Can you work these out from the model? Positions are in its coordinate system, mm. Face numbers are marked on the shaded views. A direction names the side the tool comes from. Round coordinates to 2 decimals unless told otherwise and drop trailing zeros. Write each loop counter-clockwise with the first axis right and the second up, starting at its lowest first coordinate (ties: lowest second). Pieces come first, ordered by that corner, then holes.
Q1. I'm going to push flat-ended pins straight in: pin 1 Ø5 at (y, z) = (12, 13) entering from +X; pin 2 Ø3 at (y, z) = (5, -2.5) entering from -X; pin 3 Ø5 at (y, z) = (19, 13.5) entering from -X. Where does each tip first touch, or does it pass through?
Q2. If we section it at A-A (y = 11.5): Please give me the cut outline in (x, z).
Q3. Please list where these lines run through material, in increasing order: line 1 along X through (y, z) = (16, 0); line 2 along Y through (x, z) = (19, 3); line 3 along Z through (x, y) = (-10, 17.25).
Q4. We'd pull the mould along X, two halves only. Please class the marked faces 3, 4 and 5: +X half, -X half, draft (parallel to the pull), parting line (faces both ways), or undercut.
Q5. If we section it at B-B (z = -1.5): Please give me the cut outline in (x, y), plus the area to 3 significant figures.
Q6. If we section it at C-C (x = -11.5): Please give me the cut outline in (y, z).
Q7. For the marked faces 1 and 2, which set-ups out of +Z, -Z, +X, -X, +Y, -Y let a thin tool reach every point of the face, with its end or its side?
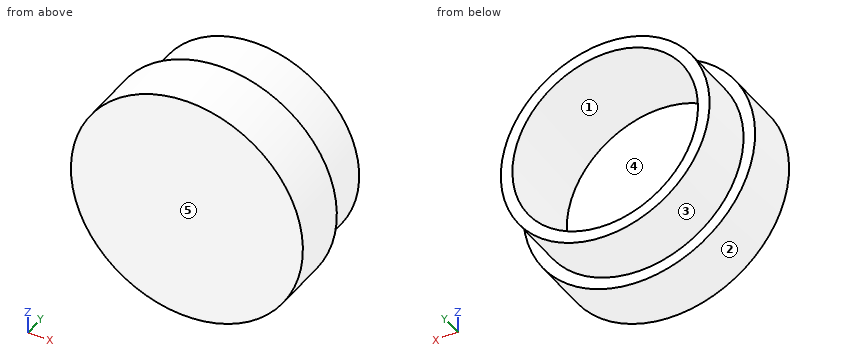
from build123d import *

# Parameters (mm, degrees)
SKETCH1_R           = 25.4
BOSS_EXTRUDE1_DEPTH = 25.4
SHELL2_T            = -5.08
CUT_EXTRUDE3_START  = -12.7
SKETCH3_R           = 25.4
SKETCH3_R_2         = 22.86
CUT_EXTRUDE3_DEPTH  = 12.7


with BuildPart() as part:
    # Sketch1 → Boss-Extrude1 (new body)
    with BuildSketch(Plane(origin=(0, 0, 0), x_dir=(1, 0, 0), z_dir=(0, 1, 0))):
        with Locations(Location((0, 0, 0), (0, 0, 270))):
            Circle(SKETCH1_R)
    extrude(amount=BOSS_EXTRUDE1_DEPTH)

    # Shell2
    shell2_openings = [part.faces().sort_by_distance(p)[0] for p in [
        (0, 25.4, 0),
    ]]
    offset(amount=SHELL2_T, openings=shell2_openings, kind=Kind.INTERSECTION)

    # Sketch3 → Cut-Extrude3 (cut)
    with BuildSketch(Plane(origin=(0, 25.4, 0), x_dir=(1, 0, 0), z_dir=(0, 1, 0)).offset(CUT_EXTRUDE3_START)):
        with Locations(Location((0, 0, 0), (0, 0, 270))):
            Circle(SKETCH3_R)
        with Locations(Location((0, 0, 0), (0, 0, 270))):
            Circle(SKETCH3_R_2, mode=Mode.SUBTRACT)
    extrude(amount=CUT_EXTRUDE3_DEPTH, mode=Mode.SUBTRACT)


solid = part.part
A:
1. pin 1: stops at x = 23.13
1. pin 2: stops at x = -25.38
1. pin 3: stops at x = -20.04
2. outline: circle Ø50.8 at (0, 0); hole circle Ø40.64 at (0, 0)
3. line 1: x = -22.86 to -20.32, 20.32 to 22.86
3. line 2: y = 0 to 5.08
3. line 3: z = -20.56 to -17.69, 17.69 to 20.56
4. face 3: parting line
4. face 4: undercut
4. face 5: draft
5. outline: (-25.36, 0) - (25.36, 0) - (25.36, 12.7) - (22.81, 12.7) - (22.81, 25.4) - (20.26, 25.4) - (20.26, 5.08) - (-20.26, 5.08) - (-20.26, 25.4) - (-22.81, 25.4) - (-22.81, 12.7) - (-25.36, 12.7) - close
5. area: 400 mm2
6. outline: (0, -22.65) - (12.7, -22.65) - (12.7, -19.76) - (25.4, -19.76) - (25.4, -16.75) - (5.08, -16.75) - (5.08, 16.75) - (25.4, 16.75) - (25.4, 19.76) - (12.7, 19.76) - (12.7, 22.65) - (0, 22.65) - close
7. face 1: +Y
7. face 2: +Y, -Y
